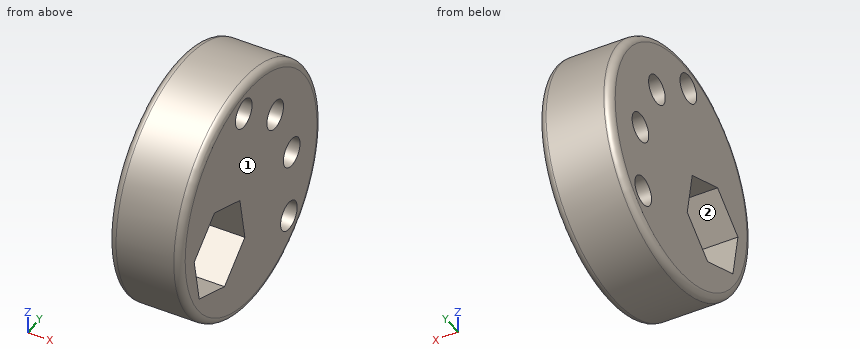
from build123d import *

# Parameters (mm, degrees)
SKIZZE1_R                       = 8.425
AUFSATZ_LINEAR_AUSTRAGEN1_DEPTH = 5
SKIZZE2_R                       = 1
SCHNITT_LINEAR_AUSTRAGEN1_DEPTH = 5
VERRUNDUNG5_R                   = 0.5
VERRUNDUNG6_R                   = 0.5


with BuildPart() as part:
    # Skizze1 → Aufsatz-Linear austragen1 (new body)
    with BuildSketch(Plane(origin=(0, 0, 0), x_dir=(0, 0, -1), z_dir=(1, 0, 0))):
        Circle(SKIZZE1_R)
    extrude(amount=AUFSATZ_LINEAR_AUSTRAGEN1_DEPTH)

    # Skizze2 → Schnitt-Linear austragen1 (cut)
    with BuildSketch(Plane(origin=(0, 0, 0), x_dir=(0, 0, -1), z_dir=(1, 0, 0))):
        with Locations((4.737160117, 4.550403752)):
            Circle(SKIZZE2_R)
        with Locations((0.175068654, 4.890321488)):
            Circle(SKIZZE2_R)
        with Locations((-3.945777315, 2.90365315)):
            Circle(SKIZZE2_R)
        with Locations((-6.521200441, -0.877275083)):
            Circle(SKIZZE2_R)
        Polygon((-0.286116888, -1.345269379), (2.887315481, -0.743416411), (4.995251626, -3.190762977), (3.929755401, -6.23996251), (0.756323031, -6.841815478), (-1.351613114, -4.394468913), align=None)
    extrude(amount=SCHNITT_LINEAR_AUSTRAGEN1_DEPTH, mode=Mode.SUBTRACT)

    # Verrundung5
    verrundung5_edges = [part.edges().sort_by_distance(p)[0] for p in [
        (5, 0, 8.425),
    ]]
    fillet(verrundung5_edges, radius=VERRUNDUNG5_R)

    # Verrundung6
    verrundung6_edges = [part.edges().sort_by_distance(p)[0] for p in [
        (0, 0, 8.425),
    ]]
    fillet(verrundung6_edges, radius=VERRUNDUNG6_R)


solid = part.part
The listing builds one solid part. Answer for the finished solid, in the listing's coordinates (mm). Face numbers are marked on the shaded views. A direction names the side the tool comes from. Coordinates: 2 decimals unless noted, no trailing zeros. Order: outer loops, then holes, each group sorted by start corner. A loop starts at its lowest first (then second) coordinate and runs counter-clockwise, first axis right, second up.
Q1. A cutting plane is placed at B-B, the plane z = 0. Write down the section's boundary in (x, y) (3 decimals).
Q2. A cutting plane is placed at A-A, the plane x = 4.2. Write down the section's boundary in (y, z) (3 decimals).
Q3. Given P1, Ø1.2, axis at y = 4.89, z = -0.18, coming from the +X side; P2, Ø3, axis at y = 2.9, z = 3.95, coming from the -X side; P3, Ø1.5, axis at x = 4.5, y = -1, coming from the +Z side; P4, Ø1, axis at x = 2, z = -2, coming from the +Y side, each flat-ended and moving along its own axis, determine where each tip first touches the part or whether it passes through.
Q4. Which of the six approach directions +Z, -Z, +X, -X, +Y, -Y give full straight-line access (tool end or side, diameter ignored) to the marked faces 1 and 2?
Q5. Consider line 1 (Z direction, x = 0.75, y = 4.75); line 2 (Y direction, x = 4.4, z = 0) (3 decimals); line 3 (Z direction, x = 1.1, y = 4.25). Determine where each line is inside the solid, lowest interval first.
Answers follow:
1. outline: (0, -7.925) arc R0.5 ccw to (0.5, -8.425) - (4.5, -8.425) arc R0.5 ccw to (5, -7.925) - (5, -5.964) - (0, -5.964) - close; (0, -1.291) - (5, -1.291) - (5, 3.906) - (0, 3.906) - close; (0, 5.875) - (5, 5.875) - (5, 7.925) arc R0.5 ccw to (4.5, 8.425) - (0.5, 8.425) arc R0.5 ccw to (0, 7.925) - close
2. outline: circle Ø16.85 at (0, 0); hole (-6.842, -0.756) - (-6.24, -3.93) - (-3.191, -4.995) - (-0.743, -2.887) - (-1.345, 0.286) - (-4.394, 1.352) - close; hole circle Ø2 at (-0.877, 6.521); hole circle Ø2 at (2.904, 3.946); hole circle Ø2 at (4.55, -4.737); hole circle Ø2 at (4.89, -0.175)
3. P1: passes through
3. P2: stops at x = 0
3. P3: stops at z = 8.42
3. P4: stops at y = 8.29
4. face 1: +Z, -Z, +X, +Y, -Y
4. face 2: +X, -X
5. line 1: z = -6.96 to -5.72, -3.76 to -1.17, 0.82 to 6.96
5. line 2: y = -8.425 to -5.964, -1.291 to 3.906, 5.875 to 8.425
5. line 3: z = -7.27 to -5.69, -3.78 to -0.94, 0.59 to 7.27
